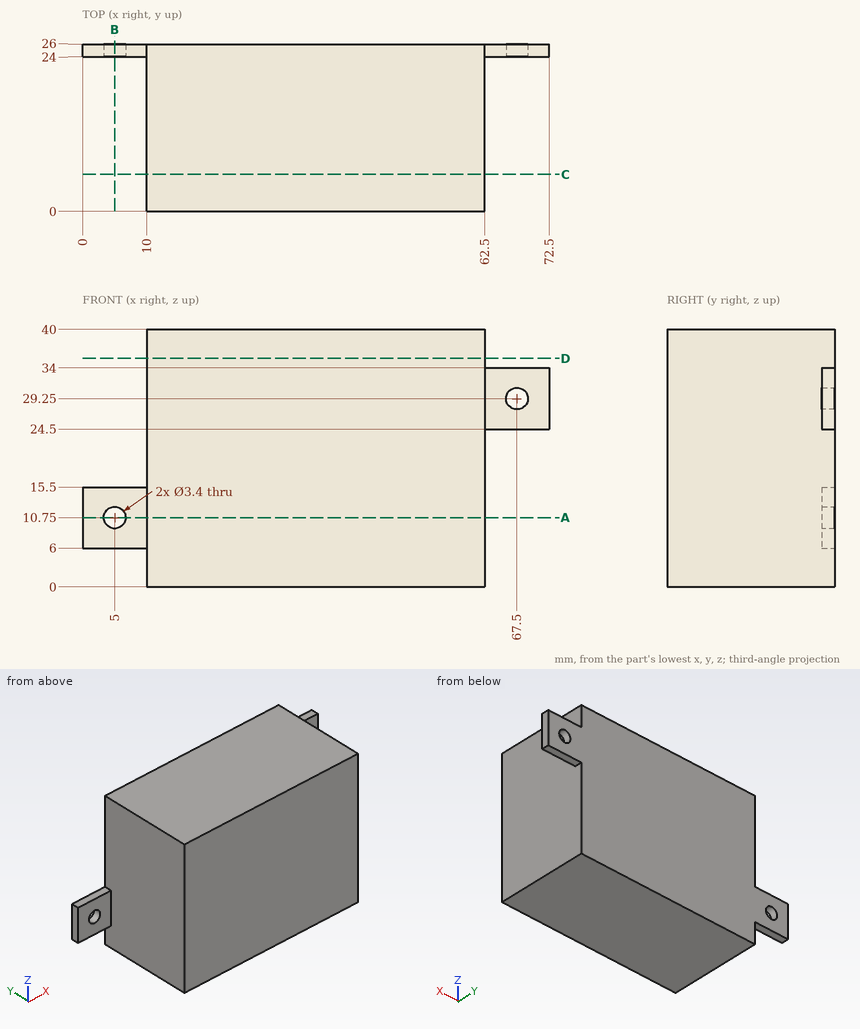
Design review of the part shown in the three views and the two pictorial views. Dimensions are in mm from the part's minimum x, y and z. Coordinates: 2 decimals unless noted, no trailing zeros. Loops run counter-clockwise (first coordinate to the right, second up) from the corner with the lowest first, then second, coordinate; pieces in that order, holes last.
(1) Consider section C-C, the plane y = 5.75. Give the boundary of the cut face in (x, z), plus the area to 3 significant figures.
Determined:
outline: (10, 0) - (62.5, 0) - (62.5, 40) - (10, 40) - close
area: 2,100 mm2
(2) Consider section D-D, the plane z = 35.5. Give the boundary of the cut face in (x, y).
Determined:
outline: (10, 0) - (62.5, 0) - (62.5, 26) - (10, 26) - close
(3) Consider section A-A, the plane z = 10.75. Give the boundary of the cut face in (x, y), plus the area to 3 significant figures.
Determined:
outline: (0, 24) - (3.3, 24) - (3.3, 26) - (0, 26) - close; (6.7, 24) - (10, 24) - (10, 0) - (62.5, 0) - (62.5, 26) - (6.7, 26) - close
area: 1,380 mm2
(4) Wall thickness on L1, parallel to Z at x = 67.5, y = 24.6; L2, parallel to X at y = 25.05, z = 29.25; L3, parallel to X at y = 24.6, z = 10.75: over which ranges is each line inside the solid? List them lowest first.
Determined:
L1: z = 24.5 to 27.55, 30.95 to 34
L2: x = 10 to 65.8, 69.2 to 72.5
L3: x = 0 to 3.3, 6.7 to 62.5
(5) Insertion check: P1, Ø12, axis at x = 19.5, z = 10, coming from the -Y side; P2, Ø1.5, axis at y = 15.5, z = 7, coming from the -X side; P3, Ø2, axis at x = 6, y = 25, coming from the +Z side; P4, Ø13, axis at y = 7, z = 17.5, coming from the +X side. Each pin has a flat end and moves straight along its axis. Give the tip position at first contact, or say it passes through.
Determined:
P1: stops at y = 0
P2: stops at x = 10
P3: stops at z = 15.5
P4: stops at x = 62.5
(6) Consider section B-B, the plane x = 5. Give the boundary of the cut face in (y, z).
Determined:
outline: (24, 6) - (26, 6) - (26, 9.05) - (24, 9.05) - close; (24, 12.45) - (26, 12.45) - (26, 15.5) - (24, 15.5) - close
